Check sheet for the drawn part. Datum: minimum x, y, z corner. Units: mm. A direction names the side the tool comes from. Give positions to 0.01 mm unless a question says otherwise; leave off trailing zeros. Loops run counter-clockwise (first coordinate to the right, second up) from the corner with the lowest first, then second, coordinate; pieces in that order, holes last. Notation, with made-up numbers: (84, 89.25) - (92, 89.25) arc R15 cw to (92, 111.25) - close; hole circle Ø2 at (43, 10.5). An arc over 180 degrees is marked (long way). Answer in a Markdown table with one row per item.
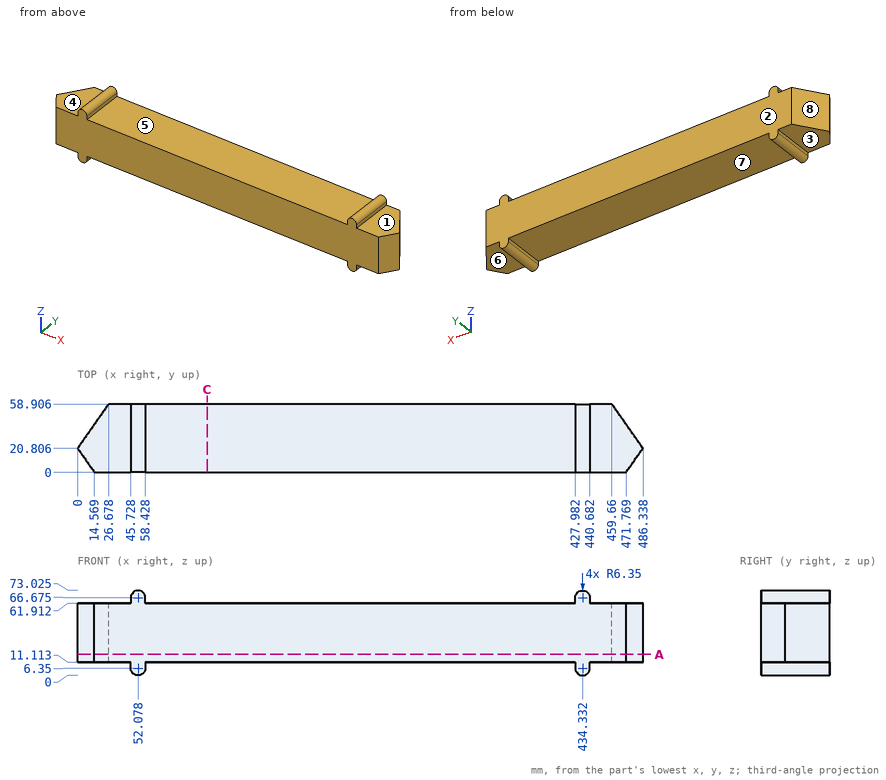
Q1. Draft check along X on the marked faces 6, 7 and 8. Enter one of: +X half, -X half, draft (parallel to the pull), parting line (faces both ways), or undercut.
Completed:
| item | result |
|---|---|
| face 6 | draft |
| face 7 | undercut |
| face 8 | -X half |
Q2. Sectioned sample at C-C (x = 111.5). Record the cut outline in (y, z).
Completed:
| item | result |
|---|---|
| outline | (0, 11.11) - (58.91, 11.11) - (58.91, 61.91) - (0, 61.91) - close |
Q3. Go/stop test with flat-tipped pins: P1, Ø6, axis at y = 36, z = 12, coming from the +X side; P2, Ø1.5, axis at x = 112.5, y = 28, coming from the -Z side; P3, Ø6, axis at x = 60, y = 48, coming from the -Z side. Record where each tip stops, or that it passes through.
Completed:
| item | result |
|---|---|
| P1 | x = 477.8 |
| P2 | z = 11.11 |
| P3 | z = 2.34 |
Q4. Tool access check on the marked faces 1, 2, 3, 4 and 5. Record the directions out of +Z, -Z, +X, -X, +Y, -Y that give a thin tool (end or side, any length) a straight path to the whole face; none if there is none.
Completed:
| item | result |
|---|---|
| face 1 | +Z, +X, +Y, -Y |
| face 2 | +Z, -Z, +X, -X, +Y |
| face 3 | -Z, -X, +Y, -Y |
| face 4 | +Z, -X, +Y, -Y |
| face 5 | +Z, +Y, -Y |
Q5. Thickness scan on line 1 (X direction, y = 24.5, z = 69.5) (1 decimal); line 2 (Z direction, x = 104, y = 51); line 3 (X direction, y = 46.5, z = 49) (1 decimal). Record the ranges inside material, lowest first.
Completed:
| item | result |
|---|---|
| line 1 | 46.4 to 57.8, 428.6 to 440 |
| line 2 | 11.11 to 61.91 |
| line 3 | 18 to 468.3 |
Q6. Sectioned sample at A-A (z = 18). Record the cut outline in (x, y).
Completed:
| item | result |
|---|---|
| outline | (0, 20.81) - (14.57, 0) - (471.77, 0) - (486.34, 20.81) - (459.66, 58.91) - (26.68, 58.91) - close |
